```python
from build123d import *

# Parameters (mm, degrees)
F1_DEPTH  = 9.398
F2_W      = 76.2
F2_H      = 33.274
F3_DEPTH  = 9.398
F4_W      = 76.2
F4_H      = 29.2016597947
F5_DEPTH  = 63.754
F6_SIZE   = 11.43
F7_W      = 76.2
F7_H      = 20.574
F8_DEPTH  = 10.414
F9_R      = 14.224
F10_DEPTH = 221.488


with BuildPart() as f1:
    # F0 (on Top) → F1 (new body)
    with BuildSketch(Plane.XY):
        Polygon((-49.3122338645, 13.7030885327), (-49.3122338645, -9.9189114673), (26.8877661355, -9.9189114673), (26.8877661355, 13.7030885327), (-6.5132338645, 59.6770885327), (-15.9112338645, 59.6770885327), align=None)
    extrude(amount=F1_DEPTH)

    # F2 (on face) → F3 (join)
    with BuildSketch(Plane.XZ.offset(9.9189114673)):
        with Locations((-11.2122338645, -16.637)):
            Rectangle(F2_W, F2_H)
    extrude(amount=-F3_DEPTH)

    # F4 (on face) → F5 (join)
    with BuildSketch(Plane.XZ.offset(9.9189114673)):
        with Locations((-11.2122338645, -18.6731701027)):
            Rectangle(F4_W, F4_H)
    extrude(amount=F5_DEPTH)

    # F6
    f6_edges = [f1.edges().sort_by_distance(p)[0] for p in [
        (26.887766, -41.795911, -4.07234),
        (-49.312234, -41.795911, -4.07234),
    ]]
    chamfer(f6_edges, length=F6_SIZE)

    # F7 (on face) → F8 (join)
    with BuildSketch(Plane(origin=(0, 0, -33.274), x_dir=(1, 0, 0), z_dir=(0, 0, -1))):
        with Locations((-11.2122338645, 31.6359114673)):
            Rectangle(F7_W, F7_H)
    extrude(amount=F8_DEPTH)

    # F9 (on face) → F10 (cut)
    with BuildSketch(Plane.XY.offset(-4.0723402053)):
        with Locations((-11.2122338645, -41.7959114673)):
            Circle(F9_R)
    extrude(amount=-F10_DEPTH, mode=Mode.SUBTRACT)


solid = f1.part
```
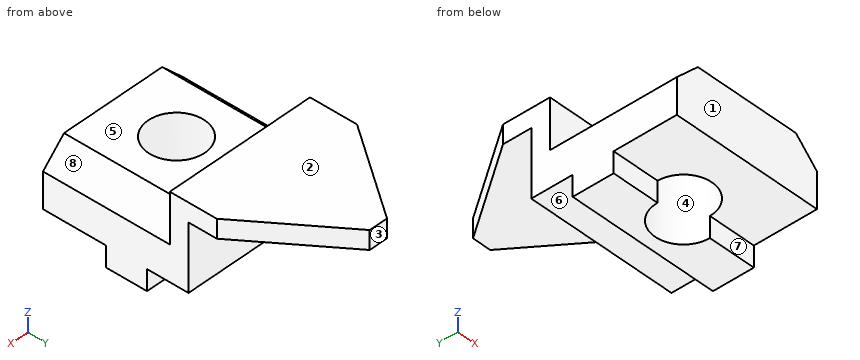
Read the model definition and answer for the solid it produces. Units are mm, in the model's axes. Face numbers are marked on the shaded views. A direction names the side the tool comes from. Round coordinates to 2 decimals unless told otherwise and drop trailing zeros. Write each loop counter-clockwise with the first axis right and the second up, starting at its lowest first coordinate (ties: lowest second). Pieces come first, ordered by that corner, then holes. Notation, with made-up numbers: (46, 59.5) - (64, 59.5) arc R6 cw to (64, 69.5) - close; hole circle Ø5 at (68.5, 8.25). An arc over 180 degrees is marked (long way). Use CSV: the item, a comma, the result in double quotes.
Q1. Find section B-B, the plane y = -37.5. Write down the section's boundary in (x, z).
Values:
outline,"(-49.31, -43.69) - (-24.77, -43.69) - (-24.77, -4.07) - (-37.88, -4.07) - (-49.31, -15.5) - close; (2.35, -43.69) - (26.89, -43.69) - (26.89, -15.5) - (15.46, -4.07) - (2.35, -4.07) - close"
Q2. Determine the mould class of the marked faces 1, 2, 3 and 4 for opening direction Y: +Y half, -Y half, draft (parallel to the pull), parting line (faces both ways), or undercut.
Values:
face 1,"-Y half"
face 2,"draft"
face 3,"+Y half"
face 4,"undercut"
Q3. Find section D-D, the plane x = 13.5. Write down the section's boundary in (y, z).
Values:
outline,"(-73.67, -33.27) - (-41.92, -33.27) - (-41.92, -43.69) - (-21.35, -43.69) - (-21.35, -33.27) - (-0.52, -33.27) - (-0.52, 0) - (32.13, 0) - (32.13, 9.4) - (-9.92, 9.4) - (-9.92, -4.07) - (-73.67, -4.07) - close"
Q4. Each of these flat-tipped pins is pushed along its axis until it touches: pin 1 Ø10 at (x, z) = (-22.5, -12) entering from +Y; pin 2 Ø6 at (x, y) = (-18.5, -9) entering from -Z; pin 3 Ø8 at (y, z) = (42.5, 4) entering from -X. Where does it stop, or does it pass through?
Values:
pin 1,"stops at y = -0.52"
pin 2,"stops at z = -33.27"
pin 3,"stops at x = -31.3"
Q5. A tool of negligible diameter and unlimited length cuts with its end or side. For the marked faces 5, 6, 7 and 8, from which of +Z, -Z, +X, -X, +Y, -Y can it reach the whole face along a straight path? Write none if from no direction.
Values:
face 5,"+Z, +X, -X, -Y"
face 6,"-Z, +X, -X, +Y"
face 7,"-Z, +X, -X, -Y"
face 8,"+Z, +X, -Y"
Q6. Find section C-C, the plane z = -8. Write down the section's boundary in (x, y).
Values:
outline,"(-49.31, -9.92) - (-41.81, -9.92) - (-41.81, -73.67) - (19.39, -73.67) - (19.39, -9.92) - (26.89, -9.92) - (26.89, -0.52) - (-49.31, -0.52) - close; hole circle Ø28.45 at (-11.21, -41.8)"
Q7. Straight lines are drawn through the part: line 1 along Y through (x, z) = (-26, -24); line 2 along Y through (x, z) = (-5.5, -21); line 3 along Y through (x, z) = (-39, -38.5). For each, find the intervals that lie inside material, in ascending order.
Values:
line 1,"y = -73.67 to -0.52"
line 2,"y = -73.67 to -54.82, -28.77 to -0.52"
line 3,"y = -41.92 to -21.35"
Q8. Find section A-A, the plane x = -14.5. Write down the section's boundary in (y, z), then the cut area to 3 significant figures.
Values:
outline,"(-73.67, -33.27) - (-55.63, -33.27) - (-55.63, -4.07) - (-73.67, -4.07) - close; (-27.96, -43.69) - (-21.35, -43.69) - (-21.35, -33.27) - (-0.52, -33.27) - (-0.52, 0) - (59.68, 0) - (59.68, 9.4) - (-9.92, 9.4) - (-9.92, -4.07) - (-27.96, -4.07) - close"
area,"2,090 mm²"
